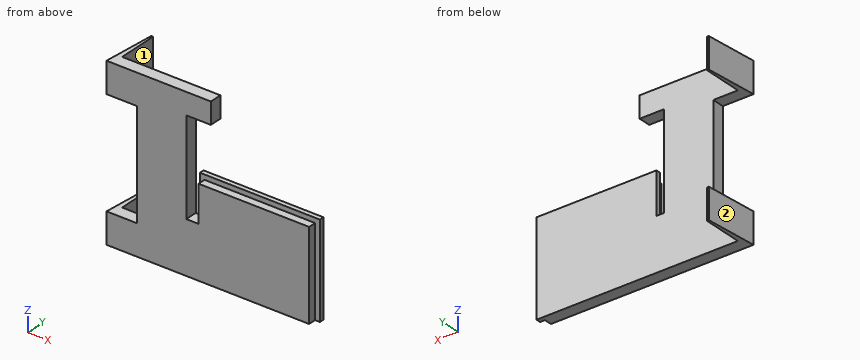
Autodesk Inventor part; units mm, degrees
ref_plane "YZ Plane" through (0, 0, 0) normal (1, 0, 0) x (0, 1, 0)
ref_plane "XZ Plane" through (0, 0, 0) normal (0, 1, 0) x (-1, 0, 0)
ref_plane "XY Plane" through (0, 0, 0) normal (0, 0, 1) x (1, 0, 0)
sketch "плоскость" plane through (0, 0, 0) normal (0, 1, 0) x (-1, 0, 0)
  line L0 (68, 55) -> (0, 55)
  line L1 (0, 55) -> (0, 0)
  line L2 (0, 0) -> (68, 0)
  line L3 (68, 0) -> (68, 55)
  dimension "d0" = 68
  dimension "d1" = 55
extrude "толщина" add sketch "плоскость" along normal blind 4
sketch "вырез" plane through (0, 4, 0) normal (0, 1, 0) x (1, 0, 0)
  line L0 (-68, 0) -> (-68, -55)
  line L1 (-68, -45) -> (-58, -45)
  line L2 (-58, -45) -> (-58, -10)
  line L3 (-58, -10) -> (-68, -10)
  line L4 (-68, -10) -> (-68, -45)
  line L5 (0, -55) -> (0, 0)
  line L6 (-68, -55) -> (0, -55)
  line L7 (0, -31) -> (-42, -31)
  line L8 (-42, -31) -> (-42, -55)
  line L9 (-42, -55) -> (0, -55)
  line L10 (0, -55) -> (0, -31)
  line L11 (0, 0) -> (-68, 0)
  point P0 (-68, -10)
  point P1 (-63, -10)
  point P2 (-63, -45)
  dimension "d4" = 35
  dimension "d5" = 10
  dimension "d25" = 58
  dimension "d34" = 10
  dimension "d35" = 10
extrude "вырез глубина" cut sketch "вырез" against normal blind 4 contours L3 L2 L1 L0
sketch "Эскиз3" plane through (0, 4, 0) normal (0, 1, 0) x (1, 0, 0)
  line L0 (-68, 0) -> (-68, -55)
  line L1 (-58, -45) -> (-68, -45)
  line L2 (-68, -55) -> (-66, -55)
  line L3 (-66, -55) -> (-66, -45)
  line L4 (-66, -45) -> (-68, -45)
  line L5 (-68, -45) -> (-68, -55)
  line L6 (-58, -10) -> (-68, -10)
  line L7 (0, 0) -> (-68, 0)
  line L8 (-68, -10) -> (-66, -10)
  line L9 (-66, -10) -> (-66, 0)
  line L10 (-66, 0) -> (-68, 0)
  line L11 (-68, 0) -> (-68, -10)
  point P0 (-68, 0)
extrude "Выдавливание3" add sketch "Эскиз3" along normal blind 13
sketch "лапки" plane through (-68, 0, 55) normal (0, 0, 1) x (1, 0, 0)
  line L0 (0, 0) -> (0, 17)
  line L1 (0, 0) -> (0, 17)
  line L2 (0, 17) -> (1.41, 17)
  line L3 (0, 0) -> (10, 0)
  line L4 (1.41, 17) -> (0, 0)
  point P0 (68, 0)
  point P1 (0, 1)
  point P2 (0, 1)
extrude "Выдавливание4" cut sketch "лапки" against normal through all
sketch "Эскиз10" plane through (0, 4, 0) normal (0, 1, 0) x (1, 0, 0)
  line L0 (0, -55) -> (0, 0)
  line L1 (-68, -55) -> (0, -55)
  line L2 (0, -31) -> (-42, -31)
  line L3 (-42, -31) -> (-42, -55)
  line L4 (-42, -55) -> (0, -55)
  line L5 (0, -55) -> (0, -31)
extrude "Выдавливание7" cut sketch "Эскиз10" against normal blind 4
sketch "Эскиз11" plane through (0, 4, 0) normal (0, 1, 0) x (1, 0, 0)
  line L0 (0, -31) -> (-42, -31)
  line L1 (-40, -17) -> (-42, -17)
  line L2 (-42, -17) -> (-42, -31)
  line L3 (-42, -31) -> (-40, -31)
  line L4 (-40, -31) -> (-40, -17)
  point P0 (0, 0)
extrude "Выдавливание8" cut sketch "Эскиз11" against normal blind 4
sketch "Эскиз12" plane through (0, 4, 0) normal (0, 1, 0) x (1, 0, 0)
  line L0 (-42, -55) -> (-42, -17)
  line L1 (-42, -48) -> (-34, -48)
  line L2 (-34, -48) -> (-34, -55)
  line L3 (-34, -55) -> (-42, -55)
  line L4 (-42, -55) -> (-42, -48)
  line L5 (-40, -31) -> (0, -31)
  point P0 (0, 0)
  point P1 (-42, -55)
  point P2 (-38, -55)
  point P3 (-38, -48)
  point P4 (-42, -51.5)
  point P5 (-34, -51.5)
  dimension "d36" = 7
  dimension "d37" = 8
  dimension "d38" = 17
extrude "Выдавливание9" add sketch "Эскиз12" against normal blind 4
sketch "Эскиз14" plane through (0, 0, 0) normal (0, -1, 0) x (1, 0, 0)
  line L0 (-42, 17) -> (-40, 17)
  line L1 (-40, 17) -> (-38, 17)
  line L2 (-38, 17) -> (-38, 31)
  line L3 (-38, 31) -> (-40, 31)
  line L4 (-40, 31) -> (-40, 17)
  line L5 (0, 31) -> (0, 0)
  line L6 (-40, 29) -> (0, 29)
  line L7 (0, 29) -> (0, 31)
  line L8 (0, 31) -> (-40, 31)
  line L9 (-40, 31) -> (-40, 29)
  line L10 (0, 0) -> (-68, 0)
  line L11 (0, 31) -> (-2, 31)
  line L12 (-2, 31) -> (-2, 0)
  line L13 (-2, 0) -> (0, 0)
  line L14 (0, 0) -> (0, 31)
  point P0 (-38, 29)
  point P1 (-2, 29)
  point P2 (-40, 24)
  point P3 (-38, 24)
  dimension "d46" = 2
  dimension "d47" = 2
  dimension "d48" = 2
extrude "Выдавливание10" cut sketch "Эскиз14" against normal blind 2.5
sketch "Эскиз15" plane through (0, 2.5, 0) normal (0, -1, 0) x (1, 0, 0)
  line L0 (-40, 31) -> (0, 31)
  line L1 (0, 0) -> (-0.4, 0)
  line L2 (-0.4, 0) -> (-0.4, 31)
  line L3 (-0.4, 31) -> (0, 31)
  line L4 (0, 31) -> (0, 0)
  line L5 (-40, 17) -> (-40, 31)
  line L6 (0, 31) -> (-40, 31)
  line L7 (-40, 31) -> (-40, 30.6)
  line L8 (-40, 30.6) -> (0, 30.6)
  line L9 (0, 30.6) -> (0, 31)
  line L10 (-38, 17) -> (-42, 17)
  line L11 (-40, 31) -> (-39.5, 31)
  line L12 (-39.5, 31) -> (-39.5, 17)
  line L13 (-39.5, 17) -> (-40, 17)
  line L14 (-40, 17) -> (-40, 31)
  point P0 (0, 31)
  point P1 (-39.5, 30.6)
  point P2 (-0.4, 30.6)
  dimension "d41" = 0.4
  dimension "d42" = 0.4
  dimension "d43" = 0.5
extrude "Выдавливание11" cut sketch "Эскиз15" against normal blind 1.5
properties part number "box_hut03_10_2025"
Build history of the part. All positions in model axes, mm. Face numbers are marked on the shaded views. A direction names the side the tool comes from. Round coordinates to 2 decimals unless told otherwise and drop trailing zeros. Write each loop counter-clockwise with the first axis right and the second up, starting at its lowest first coordinate (ties: lowest second). Pieces come first, ordered by that corner, then holes.
1) Band-saw the part on C-C, the plane y = 11.75. List the corners of the cut face in (x, z), and give its area (3 significant figures).
2) Band-saw the part on B-B, the plane x = -60. List the corners of the cut face in (y, z), and give its area (3 significant figures).
3) Drill centre lines: probe 1 along X at (y, z) = (3.5, 19); probe 2 along Y at (x, z) = (-7.5, 10); probe 3 along X at (y, z) = (2, 31). Where is each one in solid material? Low to high.
4) Band-saw the part on A-A, the plane z = 22.5. List the corners of the cut face in (x, y), and give its area (3 significant figures).
5) 3-axis set-ups, long thin cutter, end or side, ignore diameter. For the marked faces 1 and 2: which of +Z, -Z, +X, -X, +Y, -Y reach the whole face in a straight line?
6) Pin check, flat tips, straight feed: pin 1 (0.8 mm diameter, centred on y = 3, z = 21, fed in from -X); pin 2 (10 mm diameter, centred on x = -41, z = 7, fed in from +Y); pin 3 (3 mm diameter, centred on x = -26, y = 7, fed in from +Z); pin 4 (2 mm diameter, centred on y = 3, z = 51, fed in from +X). Stop position of each tip, or through.
7) Band-saw the part on D-D, the plane x = -37. List the corners of the cut face in (y, z), and give its area (3 significant figures).
Ans:
1. outline: (-67.03, 0) - (-66, 0) - (-66, 10) - (-67.03, 10) - close; (-67.03, 45) - (-66, 45) - (-66, 55) - (-67.03, 55) - close
1. area: 20.5 mm2
2. outline: (0, 0) - (4, 0) - (4, 10) - (0, 10) - close; (0, 45) - (4, 45) - (4, 55) - (0, 55) - close
2. area: 80.0 mm2
3. probe 1: x = -58 to -42, -39.5 to -0.4
3. probe 2: y = 0 to 4
3. probe 3: x = -58 to -42
4. outline: (-58, 0) - (-42, 0) - (-42, 4) - (-58, 4) - close; (-39.5, 2.5) - (-38, 2.5) - (-38, 0) - (-2, 0) - (-2, 2.5) - (-0.4, 2.5) - (-0.4, 4) - (-39.5, 4) - close
4. area: 213 mm2
5. face 1: +Z, -Z, +X, +Y
5. face 2: +Z, -Z, -X, +Y
6. pin 1: stops at x = -58
6. pin 2: stops at y = 4
6. pin 3: passes through
6. pin 4: stops at x = -34
7. outline: (0, 0) - (4, 0) - (4, 30.6) - (2.5, 30.6) - (2.5, 29) - (0, 29) - close; (0, 48) - (4, 48) - (4, 55) - (0, 55) - close
7. area: 146 mm2
